The model under review builds one solid part; all positions refer to its coordinate system, in mm. Give positions to 0.01 mm unless a question says otherwise; leave off trailing zeros. Write each loop counter-clockwise with the first axis right and the second up, starting at its lowest first coordinate (ties: lowest second). Pieces come first, ordered by that corner, then holes. Notation, with made-up numbers: (55.5, -39.75) - (99.5, -39.75) arc R10 cw to (99.5, -34.75) - close; hole circle Ø8 at (6.25, 78.5). An arc over 180 degrees is marked (long way). Write item = value, one per line.
```python
from build123d import *

# Parameters (mm, degrees)
SKETCH1_W           = 250.825
SKETCH1_H           = 203.2
SKETCH1_R           = 1.5875
BOSS_EXTRUDE1_DEPTH = 1.5875
SKETCH2_W           = 14.2875
SKETCH2_H           = 139.7
SKETCH2_W_2         = 1.5875
SKETCH2_H_2         = 133.35
SKETCH2_W_3         = 88.9
SKETCH2_H_3         = 9.525
SKETCH2_W_4         = 85.725
SKETCH2_H_4         = 1.5875
BOSS_EXTRUDE2_DEPTH = 6.35


with BuildPart() as part:
    # Sketch1 → Boss-Extrude1 (new body)
    with BuildSketch(Plane(origin=(0, 0, 0), x_dir=(1, 0, 0), z_dir=(0, 1, 0))):
        with Locations((125.4125, 101.6)):
            Rectangle(SKETCH1_W, SKETCH1_H)
        with Locations(Location((31.75, 196.85, 0), (0, 0, 270))):
            Circle(SKETCH1_R, mode=Mode.SUBTRACT)
        with Locations(Location((165.1, 196.85, 0), (0, 0, 270))):
            Circle(SKETCH1_R, mode=Mode.SUBTRACT)
        with Locations(Location((238.252, 196.85, 0), (0, 0, 270))):
            Circle(SKETCH1_R, mode=Mode.SUBTRACT)
        with Locations(Location((238.252, 38.1, 0), (0, 0, 270))):
            Circle(SKETCH1_R, mode=Mode.SUBTRACT)
        with Locations(Location((190.5, 34.925, 0), (0, 0, 270))):
            Circle(SKETCH1_R, mode=Mode.SUBTRACT)
        with Locations(Location((9.525, 38.1, 0), (0, 0, 270))):
            Circle(SKETCH1_R, mode=Mode.SUBTRACT)
        with Locations(Location((57.15, 166.6875, 0), (0, 0, 270))):
            Circle(SKETCH1_R, mode=Mode.SUBTRACT)
        with Locations(Location((131.7625, 166.6875, 0), (0, 0, 270))):
            Circle(SKETCH1_R, mode=Mode.SUBTRACT)
        with Locations(Location((131.7625, 92.075, 0), (0, 0, 270))):
            Circle(SKETCH1_R, mode=Mode.SUBTRACT)
        with Locations(Location((57.15, 92.075, 0), (0, 0, 270))):
            Circle(SKETCH1_R, mode=Mode.SUBTRACT)
    extrude(amount=BOSS_EXTRUDE1_DEPTH)

    # Sketch2 → Boss-Extrude2 (add)
    # profile 1 of 3: a face of its own
    with BuildSketch(Plane(origin=(0, 1.5875, 0), x_dir=(1, 0, 0), z_dir=(0, 1, 0))):
        with Locations((151.60625, 127)):
            Rectangle(SKETCH2_W, SKETCH2_H)
        with Locations((148.034375, 127)):
            Rectangle(SKETCH2_W_2, SKETCH2_H_2, mode=Mode.SUBTRACT)
        with Locations((155.178125, 127)):
            Rectangle(SKETCH2_W_2, SKETCH2_H_2, mode=Mode.SUBTRACT)
    # profile 2 of 3: a face of its own
    with BuildSketch(Plane(origin=(0, 1.5875, 0), x_dir=(1, 0, 0), z_dir=(0, 1, 0))):
        with Locations((177.00625, 117.475)):
            Rectangle(SKETCH2_W, SKETCH2_H)
        with Locations((173.434375, 117.475)):
            Rectangle(SKETCH2_W_2, SKETCH2_H_2, mode=Mode.SUBTRACT)
        with Locations((180.578125, 117.475)):
            Rectangle(SKETCH2_W_2, SKETCH2_H_2, mode=Mode.SUBTRACT)
    # profile 3 of 3: a face of its own
    with BuildSketch(Plane(origin=(0, 1.5875, 0), x_dir=(1, 0, 0), z_dir=(0, 1, 0))):
        with Locations((87.3125, 20.6375)):
            Rectangle(SKETCH2_W_3, SKETCH2_H_3)
        with Locations((87.3125, 21.43125)):
            Rectangle(SKETCH2_W_4, SKETCH2_H_4, mode=Mode.SUBTRACT)
    extrude(amount=BOSS_EXTRUDE2_DEPTH)


solid = part.part
```
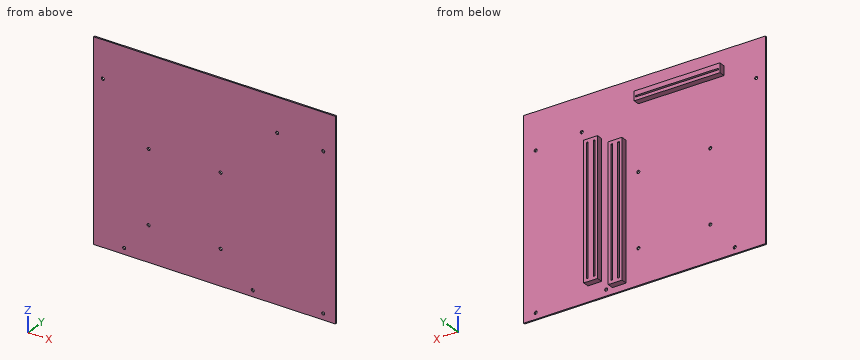
1. For line 1 (X direction, y = 4.75, z = -141); line 2 (X direction, y = 0.8, z = -38.1) (1 decimal); line 3 (Z direction, x = 81.5, y = 4.5) (1 decimal), list the stretches that pass through material, from the lowest coordinate up. Write a range as from..to.
Findings below:
line_1 = 144.46..147.24, 148.83..154.38, 155.97..158.75, 169.86..172.64, 174.23..179.78, 181.37..184.15
line_2 = 0..7.9, 11.1..236.7, 239.8..250.8
line_3 = -25.4..-22.2, -20.6..-15.9
2. Take a section at D-D on x = 204.5. Give the boundary of the cut face in (y, z).
Findings below:
outline = (0, -203.2) - (1.59, -203.2) - (1.59, 0) - (0, 0) - close
3. Take a section at C-C on x = 104. Give the boundary of the cut face in (y, z) (1 decimal), and give its area (3 significant figures).
Findings below:
outline = (0, -203.2) - (1.6, -203.2) - (1.6, -25.4) - (7.9, -25.4) - (7.9, -22.2) - (1.6, -22.2) - (1.6, -20.6) - (7.9, -20.6) - (7.9, -15.9) - (1.6, -15.9) - (1.6, 0) - (0, 0) - close
area = 373 mm²
4. Insertion check: P1, Ø0.8, axis at y = 4, z = -21.5, coming from the +X side; P2, Ø1.5, axis at x = 165.5, z = -45.5, coming from the +Y side; P3, Ø1.9, axis at x = 102.5, y = 5, coming from the -Z side; P4, Ø1.9, axis at x = 238.252, z = -196.85, coming from the +Y side. Each pin has a flat end and moves straight along its axis. Give the tip position at first contact, or say it passes through.
Findings below:
P1 = 131.76
P2 = 1.59
P3 = -25.4
P4 = through
5. Take a section at A-A on y = 5. Count the separate pieces of the cut face and the enclosed holes in it, and give its area (3 significant figures).
Findings below:
separate_pieces = 3
enclosed_holes = 5
area = 3,860 mm²
